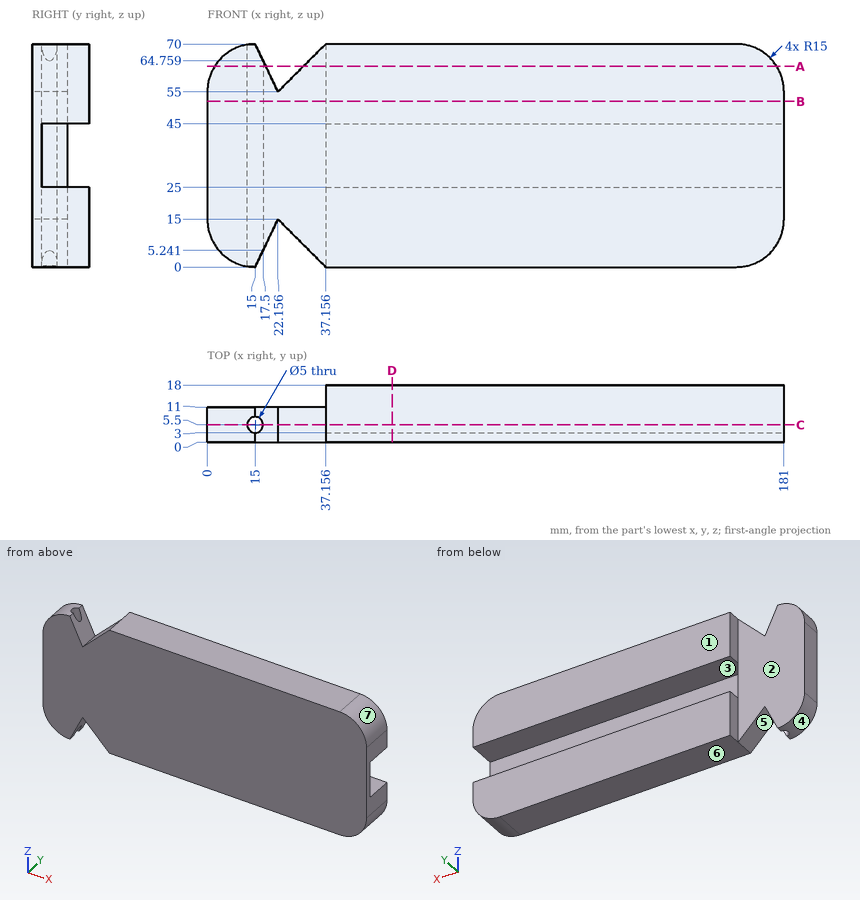
Geometry: see drawing. Coordinates: mm, zero at the bounding-box minimum. A direction names the side the tool comes from. Coordinates: 2 decimals unless noted, no trailing zeros. Write each loop counter-clockwise with the first axis right and the second up, starting at its lowest first coordinate (ties: lowest second). Pieces come first, ordered by that corner, then holes. Notation, with made-up numbers: M 4,56 L 33,56 A16 ccw 33,63 Z; hole C 63.5,-26.5 d7. An arc over 180 degrees is marked long. Answer as a JSON object with one key per item and string values.
1. Contact query for flat-ended pins moving along their axis: P1, Ø1, axis at y = 5.5, z = 36.5, coming from the +X side; P2, Ø7.5, axis at y = 14.5, z = 7, coming from the -X side (1 decimal); P3, Ø2, axis at y = 13, z = 56.5, coming from the -X side. Output: stop coordinate, or through.
Evaluation:
{"P1": "x = 37.16", "P2": "x = 1.6", "P3": "x = 37.16"}
2. Cut plane A-A on z = 63. Output: boundary loops of the cut face in (x, y) (1 decimal).
Evaluation:
{"outline": "M 2.3,0 L 18.3,0 L 18.3,11 L 2.3,11 Z; M 30.2,0 L 178.7,0 L 178.7,18 L 37.2,18 L 37.2,11 L 30.2,11 Z; hole C 15,5.5 d5"}
3. Access query for the marked faces 1, 2 and 3. Directions: +Z, -Z, +X, -X, +Y, -Y. A direction counts if a zero-diameter tool reaches every point of the face in a straight line with its end or side. Return the directions, or none.
Evaluation:
{"face 1": "+Z, -Z, +X, -X, +Y", "face 2": "+Z, -Z, -X, +Y", "face 3": "+X, +Y"}
4. Cut plane D-D on x = 58. Output: boundary loops of the cut face in (y, z).
Evaluation:
{"outline": "M 0,0 L 18,0 L 18,25 L 3,25 L 3,45 L 18,45 L 18,70 L 0,70 Z"}
5. Ray query, L1, parallel to Z at x = 123.5, y = 16.75; L2, parallel to X at y = 7.5, z = 4 (1 decimal); L3, parallel to X at y = 5.75, z = 40 (1 decimal). Return the intervals inside material, ascending.
Evaluation:
{"L1": "0 to 25, 45 to 70", "L2": "4.8 to 13.5, 16.5 to 16.9, 33.2 to 176.2", "L3": "0 to 12.5, 17.5 to 37.2"}
6. Draft query along X for the marked faces 4, 5, 6 and 7. Return one class per face: released by +X, released by -X, zero draft, split by the parting line, or undercut.
Evaluation:
{"face 4": "released by -X", "face 5": "undercut", "face 6": "zero draft", "face 7": "released by +X"}
7. Cut plane C-C on y = 5.5. Output: boundary loops of the cut face in (x, z) (1 decimal), plus the area to 3 significant figures.
Evaluation:
{"outline": "M 0,15 A15 ccw 12.5,0.2 L 12.5,69.8 A15 ccw 0,55 Z; M 17.5,5.2 L 22.2,15 L 37.2,0 L 166,0 A15 ccw 181,15 L 181,25 L 37.2,25 L 37.2,45 L 181,45 L 181,55 A15 ccw 166,70 L 37.2,70 L 22.2,55 L 17.5,64.8 Z", "area": "8,930 mm^2"}
8. Cut plane B-B on z = 52. Output: boundary loops of the cut face in (x, y) (1 decimal), plus the area to 3 significant figures.
Evaluation:
{"outline": "M 0,0 L 181,0 L 181,18 L 37.2,18 L 37.2,11 L 0,11 Z; hole C 15,5.5 d5", "area": "2,980 mm^2"}
